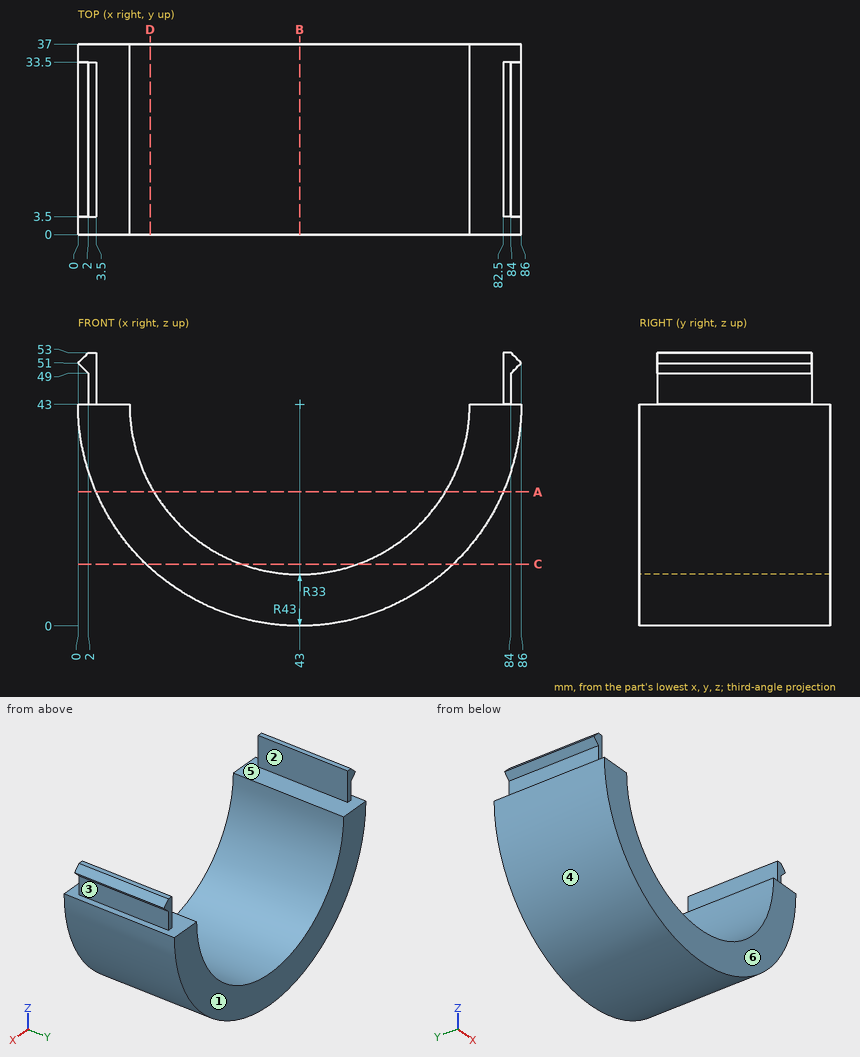
Geometry check sheet. Reference: drawing and pictorial views, mm from the part's lowest x, y, z. A direction names the side the tool comes from. Give positions to 0.01 mm unless a question says otherwise; leave off trailing zeros. Write each loop counter-clockwise with the first axis right and the second up, starting at its lowest first coordinate (ties: lowest second). Pieces come first, ordered by that corner, then holes. Notation, with made-up numbers: (86.5, 46.5) -> (91.5, 46.5) arc R26 cw to (91.5, 79.5) -> close; hole circle Ø4 at (42, 46.25). An arc over 180 degrees is marked (long way). One line per item, written item: value. Start each with the question number.
Item 1: Section check C-C on z = 12. Record the cut outline in (x, y), then the cut area to 3 significant figures.
Item 2: Material ranges on probe 1 along X at (y, z) = (12, 21.5); probe 2 along X at (y, z) = (20.5, 22); probe 3 along Z at (x, y) = (53.5, 33.5), recorded low to high. Write a range as from..to.
Item 3: Section check A-A on z = 26. Record the cut outline in (x, y), then the cut area to 3 significant figures.
Item 4: Draft check along Z on the marked faces 3, 4, 5 and 6. Enter one of: +Z half, -Z half, draft (parallel to the pull), parting line (faces both ways), or undercut.
Item 5: Section check D-D on x = 14. Record the cut outline in (y, z), then the cut area to 3 significant figures.
Item 6: Gauge pin test, flat ends, axial feed: pin 1 (3 mm diameter, centred on x = 6.5, y = 21, fed in from +Z); pin 2 (1.8 mm diameter, centred on x = 85, z = 48, fed in from -Y); pin 3 (1.8 mm diameter, centred on x = 1.5, z = 49.5, fed in from +Y); pin 4 (12 mm diameter, centred on y = 18, z = 18, fed in from -X). Record the tip position at first contact, or that the pin passes through.
Item 7: Tool access check on the marked faces 1 and 2. Record the directions out of +Z, -Z, +X, -X, +Y, -Y that give a thin tool (end or side, any length) a straight path to the whole face; none if there is none.
Item 8: Section check B-B on x = 43. Record the cut outline in (y, z).
Results list:
1. outline: (13.2, 0) -> (31.69, 0) -> (31.69, 37) -> (13.2, 37) -> close; (54.31, 0) -> (72.8, 0) -> (72.8, 37) -> (54.31, 37) -> close
1. area: 1,370 mm²
2. probe 1: 5.76..17.97, 68.03..80.24
2. probe 2: 5.48..17.54, 68.46..80.52
2. probe 3: 1.3..11.72
3. outline: (3.5, 0) -> (14.72, 0) -> (14.72, 37) -> (3.5, 37) -> close; (71.28, 0) -> (82.5, 0) -> (82.5, 37) -> (71.28, 37) -> close
3. area: 830 mm²
4. face 3: undercut
4. face 4: -Z half
4. face 5: undercut
4. face 6: draft
5. outline: (0, 11.25) -> (37, 11.25) -> (37, 27.25) -> (0, 27.25) -> close
5. area: 592 mm²
6. pin 1: z = 43
6. pin 2: through
6. pin 3: y = 33.5
6. pin 4: x = 4.43
7. face 1: +Z, -Z, +X, -X, +Y
7. face 2: +Z, +Y, -Y
8. outline: (0, 0) -> (37, 0) -> (37, 10) -> (0, 10) -> close
